```python
from build123d import *

# Parameters (mm, degrees)
F0_R     = 36.1810919244
F1_DEPTH = 25.4
F2_DEPTH = 25.4
F3_DEPTH = 90.17


with BuildPart() as f1:
    # F0 (on Front) → F1 (new body)
    with BuildSketch(Plane.XZ):
        with Locations((-101.2930572033, 34.8807759583)):
            Circle(F0_R)
    extrude(amount=F1_DEPTH)

    # F2 (add): faces of the model
    f2_faces = [f1.faces().sort_by_distance(p)[0] for p in [
        (-101.2930572033, -25.4, 34.8807759583),
        (-101.2930572033, 0, 34.8807759583),
    ]]
    extrude(f2_faces, amount=F2_DEPTH, dir=(0, -1, 0))

    # F3 (add): faces of the model
    f3_faces = [f1.faces().sort_by_distance(p)[0] for p in [
        (-101.2930572033, -50.8, 34.8807759583),
        (-101.2930572033, 0, 34.8807759583),
    ]]
    extrude(f3_faces, amount=F3_DEPTH, dir=(0, -1, 0))


solid = f1.part
```
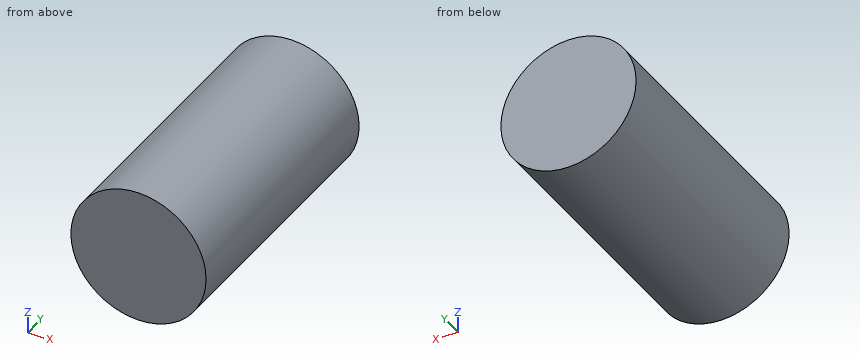
Check sheet for the modelled part. Datum: model origin and axes. Units: mm. Coordinates: 2 decimals unless noted, no trailing zeros. Loops run counter-clockwise (first coordinate to the right, second up) from the corner with the lowest first, then second, coordinate; pieces in that order, holes last.
1) Sectioned sample at A-A (x = -111). Record the boundary of the cut face in (y, z).
2) Gauge pin test, flat ends, axial feed: pin 1 (5 mm diameter, centred on x = -83.5, y = -108, fed in from -Z); pin 2 (4 mm diameter, centred on y = -119.5, z = 17.5, fed in from +X); pin 3 (5 mm diameter, centred on x = -99, y = -122, fed in from -Z). Record the tip position at first contact, or that the pin passes through.
3) Sectioned sample at C-C (y = -16.5). Record the boundary of the cut face in (x, z).
4) Sectioned sample at B-B (z = 62). Record the boundary of the cut face in (x, y).
5) Material ranges on probe 1 along X at (y, z) = (-18.5, 35); probe 2 along Z at (x, y) = (-88.5, -45); probe 3 along X at (y, z) = (-60.5, 53), recorded low to high.
Check sheet entries:
1. outline: (-140.97, 0.03) - (0, 0.03) - (0, 69.74) - (-140.97, 69.74) - close
2. pin 1: stops at z = 2.09
2. pin 2: stops at x = -68.54
2. pin 3: stops at z = -1.3
3. outline: circle Ø72.36 at (-101.29, 34.88)
4. outline: (-125.24, -140.97) - (-77.34, -140.97) - (-77.34, 0) - (-125.24, 0) - close
5. probe 1: x = -137.47 to -65.11
5. probe 2: z = 1.04 to 68.72
5. probe 3: x = -132.61 to -69.98
